Work out the finished part from the listing and answer in its coordinate system (mm). A direction names the side the tool comes from. Coordinates: 2 decimals unless noted, no trailing zeros. Loops run counter-clockwise (first coordinate to the right, second up) from the corner with the lowest first, then second, coordinate; pieces in that order, holes last. Notation, with made-up numbers: (87.5, 23.5) -> (137.5, 23.5) arc R23 ccw to (137.5, 31.5) -> close; hole circle Ø11 at (47.5, -32). An arc over 180 degrees is marked (long way). Use a Markdown table: item, result. Add a question column.
```python
from build123d import *

# Parameters (mm, degrees)
SKETCH1_W           = 50.8
SKETCH1_H           = 50.8
BOSS_EXTRUDE1_DEPTH = 25.4
SKETCH2_R           = 7.9375
CUT_EXTRUDE1_DEPTH  = 25.4
SKETCH4_R           = 14.80168028
CUT_EXTRUDE2_DEPTH  = 113.055003212


with BuildPart() as part:
    # Sketch1 → Boss-Extrude1 (new body)
    with BuildSketch(Plane.XY):
        with Locations((25.4, 25.4)):
            Rectangle(SKETCH1_W, SKETCH1_H)
    extrude(amount=BOSS_EXTRUDE1_DEPTH)

    # Sketch2 → Cut-Extrude1 (cut)
    with BuildSketch(Plane(origin=(50.8, 0, 0), x_dir=(0, 0, -1), z_dir=(1, 0, 0))):
        with Locations((-12.7, 25.4)):
            Circle(SKETCH2_R)
    extrude(amount=-CUT_EXTRUDE1_DEPTH, mode=Mode.SUBTRACT)

    # Sketch4 → Cut-Extrude2 (cut, through all)
    with BuildSketch(Plane(origin=(-43.536509722, 0, 32.807113228), x_dir=(0, 1, 0), z_dir=(-0.7986355100472856, 0, 0.6018150231520579))):
        with Locations(Location((25.4, -29.09758227, 0), (0, 0, 237.964118951))):
            Circle(SKETCH4_R)
    extrude(amount=-CUT_EXTRUDE2_DEPTH, mode=Mode.SUBTRACT)


solid = part.part
```
Item 1: Section A-A (y = 11.5) is taken. Determine the outline of the cut face in (x, z).
Item 2: Given pin 1 (5 mm diameter, centred on x = 6, z = 22, fed in from -Y); pin 2 (6 mm diameter, centred on y = 28, z = 8, fed in from +X), each flat-ended and moving along its own axis, determine where each tip first touches the part or whether it passes through.
Item 3: Section B-B (y = 22.5) is taken. Determine the outline of the cut face in (x, z), then the cut area to 3 significant figures.
Item 4: Find the intervals of material crossed by probe 1 along Y at (x, z) = (39, 5.5); probe 2 along Y at (x, z) = (29.5, 22.25); probe 3 along X at (y, z) = (13.5, 18), in increasing order.
Item 5: Section C-C (y = 35.5) is taken. Determine the outline of the cut face in (x, z).
Item 6: For faces 5 (the face through (25, 50.8, 13)), 6 (the face through (48.795, 25.558, 20.636)), determine the directions among +Z, -Z, +X, -X, +Y, -Y from which every point of the face is accessible in a straight line to the end or side of a thin tool.
Item 7: For a pull along X with two mould halves and no side action, classify faces 1 (the face through (19, 26, 0)), 2 (the face through (0, 25, 13)), 3 (the face through (50.8, 25, 21)), 4 (the face through (18.428, 23.996, 4.098)) as +X half, -X half, draft (parallel to the pull), parting line (faces both ways), or undercut.
Output:
| question | item | result |
|---|---|---|
| 1 | outline | (0, 0) -> (39.9, 0) -> (6.19, 25.4) -> (0, 25.4) -> close; (23.1, 25.4) -> (50.8, 4.52) -> (50.8, 25.4) -> close |
| 2 | pin 1 | stops at y = 0 |
| 2 | pin 2 | stops at x = 17.63 |
| 3 | outline | (0, 0) -> (24.23, 0) -> (0, 18.26) -> close; (38.76, 25.4) -> (45.81, 20.09) -> (50.8, 20.09) -> (50.8, 25.4) -> close |
| 3 | area | 266 mm2 |
| 4 | probe 1 | y = 0 to 10.65, 40.15 to 50.8 |
| 4 | probe 2 | y = 0 to 12.07, 38.73 to 50.8 |
| 4 | probe 3 | x = 0 to 9.84, 39.09 to 50.8 |
| 5 | outline | (0, 0) -> (30.37, 0) -> (0, 22.89) -> close; (32.62, 25.4) -> (50.8, 11.7) -> (50.8, 25.4) -> close |
| 6 | face 5 | +Z, -Z, +X, -X, +Y |
| 6 | face 6 | -Z, +X |
| 7 | face 1 | draft |
| 7 | face 2 | -X half |
| 7 | face 3 | +X half |
| 7 | face 4 | undercut |
